Autodesk Inventor part; units mm, degrees
ref_plane "rail_to_adjusting_block_XY" through (0, 0, -30) normal (0, 1, 0) x (1, 0, 0)
ref_plane "rail_to_adjusting_block_YZ" through (0, 0, -30) normal (1, 0, 0) x (0, 0, -1)
ref_plane "rail_to_adjusting_block_ZX" through (0, 0, -30) normal (0, 0, -1) x (0, 1, 0)
sketch "Sketch_12" plane through (0, 0, 0) normal (0, 0, 1) x (1, 0, 0)
  line L0 (-2.5, 3.7) -> (-2.5, 3.1084)
  line L1 (-2.5, 3.1084) -> (-2.3242, 3.0098)
  arc A0 (-2.1007, 2.75) -> (-2.3242, 3.0098) centre (-2.5686, 2.5736) ccw
  line L2 (-2.1007, 2.75) -> (-1.5, 2.75)
  line L3 (-1.5, 2.75) -> (-1.5, 2.25)
  line L4 (-1.5, 2.25) -> (-2.1007, 2.25)
  arc A1 (-2.3242, 1.9902) -> (-2.1007, 2.25) centre (-2.5686, 2.4264) ccw
  line L5 (-2.3242, 1.9902) -> (-2.5, 1.8917)
  line L6 (-2.5, 1.8917) -> (-2.5, 0.3)
  line L7 (-2.5, 0.3) -> (-2.2, 0)
  line L8 (-2.2, 0) -> (2.2, 0)
  line L9 (2.2, 0) -> (2.5, 0.3)
  line L10 (2.5, 0.3) -> (2.5, 1.8917)
  line L11 (2.5, 1.8917) -> (2.3242, 1.9902)
  arc A2 (2.1007, 2.25) -> (2.3242, 1.9902) centre (2.5686, 2.4263) ccw
  line L12 (2.1007, 2.25) -> (1.5, 2.25)
  line L13 (1.5, 2.25) -> (1.5, 2.75)
  line L14 (1.5, 2.75) -> (2.1007, 2.75)
  arc A3 (2.3242, 3.0098) -> (2.1007, 2.75) centre (2.5686, 2.5737) ccw
  line L15 (2.3242, 3.0098) -> (2.5, 3.1084)
  line L16 (2.5, 3.1084) -> (2.5, 3.7)
  line L17 (2.5, 3.7) -> (2.2, 4)
  line L18 (2.2, 4) -> (-2.2, 4)
  line L19 (-2.2, 4) -> (-2.5, 3.7)
extrude "Extrusion1" add sketch "Sketch_12" along normal mid plane 70
sketch "Sketch2" plane through (-2.2, 4, 35) normal (0, 1, 0) x (1, 0, 0)
  point P0 (2.2, 65)
hole "Hole1" at (0, 4, -30) direction (0, -1, 0) diameter 2.4 depth 4 counterbore diameter 3.5 counterbore depth 1
pattern_linear "Rectangular Pattern1" count 5 spacing 15 along (0, 0, 1) of "Hole1"
ref_plane "rail_to_adjusting_block_XY" through (0, 0, -30) normal (0, 1, 0) x (1, 0, 0)
ref_plane "rail_to_adjusting_block_YZ" through (0, 0, -30) normal (1, 0, 0) x (0, 0, -1)
ref_plane "rail_to_adjusting_block_ZX" through (0, 0, -30) normal (0, 0, -1) x (0, 1, 0)
ref_plane "screw_1_XY" through (0, 3, 30) normal (0, -1, 0) x (1, 0, 0)
ref_plane "screw_1_YZ" through (0, 3, 30) normal (1, 0, 0) x (0, 0, 1)
ref_plane "screw_1_ZX" through (0, 3, 30) normal (0, 0, 1) x (0, -1, 0)
ref_plane "screw_2_XY" through (0, 3, 15) normal (0, -1, 0) x (1, 0, 0)
ref_plane "screw_2_YZ" through (0, 3, 15) normal (1, 0, 0) x (0, 0, 1)
ref_plane "screw_2_ZX" through (0, 3, 15) normal (0, 0, 1) x (0, -1, 0)
ref_plane "screw_3_XY" through (0, 3, 0) normal (0, -1, 0) x (1, 0, 0)
ref_plane "screw_3_YZ" through (0, 3, 0) normal (1, 0, 0) x (0, 0, 1)
ref_plane "screw_3_ZX" through (0, 3, 0) normal (0, 0, 1) x (0, -1, 0)
ref_plane "screw_4_XY" through (0, 3, -15) normal (0, -1, 0) x (1, 0, 0)
ref_plane "screw_4_YZ" through (0, 3, -15) normal (1, 0, 0) x (0, 0, 1)
ref_plane "screw_4_ZX" through (0, 3, -15) normal (0, 0, 1) x (0, -1, 0)
ref_plane "screw_5_XY" through (0, 3, -30) normal (0, -1, 0) x (1, 0, 0)
ref_plane "screw_5_YZ" through (0, 3, -30) normal (1, 0, 0) x (0, 0, 1)
ref_plane "screw_5_ZX" through (0, 3, -30) normal (0, 0, 1) x (0, -1, 0)
ref_plane "to_block_XY" through (0, 4, 17.5) normal (0, 0, 1) x (1, 0, 0)
ref_plane "to_block_YZ" through (0, 4, 17.5) normal (1, 0, 0) x (0, 1, 0)
ref_plane "to_block_ZX" through (0, 4, 17.5) normal (0, 1, 0) x (0, 0, 1)
ref_plane "to_block_2_XY" through (0, 4, -17.5) normal (0, 0, 1) x (1, 0, 0)
ref_plane "to_block_2_YZ" through (0, 4, -17.5) normal (1, 0, 0) x (0, 1, 0)
ref_plane "to_block_2_ZX" through (0, 4, -17.5) normal (0, 1, 0) x (0, 0, 1)
ref_plane "to_kue_XY" through (0, 0, 0) normal (0, 1, 0) x (1, 0, 0)
ref_plane "to_kue_YZ" through (0, 0, 0) normal (1, 0, 0) x (0, 0, -1)
ref_plane "to_kue_ZX" through (0, 0, 0) normal (0, 0, -1) x (0, 1, 0)
properties part number "SSE2B6-70_r"
Can you work these out from the model? Positions are in its coordinate system, mm. A direction names the side the tool comes from. Give positions to 0.01 mm unless a question says otherwise; leave off trailing zeros. Loops run counter-clockwise (first coordinate to the right, second up) from the corner with the lowest first, then second, coordinate; pieces in that order, holes last. Notation, with made-up numbers: M -15.5,27 L 7.5,27 A31 ccw 7.5,63 Z; hole C 39.5,-35 d3. An arc over 180 degrees is marked long. One line per question, with ' | ' between items. Start each with the question number.
Q1. If we mould it in two halves opening along X, with no side actions, what happens to faces 1 (the cylindrical face through (-0.526, 3.493, -13.331)), 2 (the flat face through (-2.5, 1, 0)), 3 (the flat face through (-1.5, 0, -0.5))? For each: +X half, -X half, draft (parallel to the pull), parting line (faces both ways), or undercut.
Q2. For pin 1 Ø1.9 at (x, z) = (0, 30) entering from +Y; pin 2 Ø3 at (x, z) = (0.5, -14.5) entering from +Y, each with a flat end and sliding along its axis, tell me the tip position at first contact or that it passes through.
Q3. For faces 4 (the flat face through (0, 2, -35)), 5 (the cylindrical face through (-0.08, 3.49, 28.25)), which set-ups out of +Z, -Z, +X, -X, +Y, -Y let a thin tool reach every point of the face, with its end or its side?
Q4. If I drill on line 1 (Z direction, x = 0, y = 1.55); line 2 (Y direction, x = -1.7, z = 26); line 3 (Z direction, x = -0.95, y = 0.65), over which ranges is the centre line in solid material (lowest first)? Write a range as from..to.
Q5. If we section it at B-B (z = 25.5): Please give me the cut outline in (x, y).
Q6. If we section it at C-C (x = 0): State how many separate pieces and enclosed holes the cut face has, plus the area to 4 significant figures.
Computed:
1) face 1: undercut | face 2: -X half | face 3: draft
2) pin 1: passes through | pin 2: stops at y = 4
3) face 4: -Z, +X, -X, +Y, -Y | face 5: +Y
4) line 1: z = -35..-31.2, -28.8..-16.2, -13.8..-1.2, 1.2..13.8, 16.2..28.8, 31.2..35 | line 2: y = 0..2.25, 2.75..4 | line 3: z = -35..-30.73, -29.27..-15.73, -14.27..-0.73, 0.73..14.27, 15.73..29.27, 30.73..35
5) outline: M -2.5,0.3 L -2.2,0 L 2.2,0 L 2.5,0.3 L 2.5,1.89 L 2.32,1.99 A0.5 cw 2.1,2.25 L 1.5,2.25 L 1.5,2.75 L 2.1,2.75 A0.5 cw 2.32,3.01 L 2.5,3.11 L 2.5,3.7 L 2.2,4 L -2.2,4 L -2.5,3.7 L -2.5,3.11 L -2.32,3.01 A0.5 cw -2.1,2.75 L -1.5,2.75 L -1.5,2.25 L -2.1,2.25 A0.5 cw -2.32,1.99 L -2.5,1.89 Z
6) separate pieces: 6 | enclosed holes: 0 | area: 226.5 mm²
